from build123d import *

# Parameters (mm, degrees)
SKETCH1_W           = 23
SKETCH1_H           = 12
BOSS_EXTRUDE1_DEPTH = 4
SKETCH2_R           = 1.5
CUT_EXTRUDE1_DEPTH  = 10
SKETCH3_R           = 2
CUT_EXTRUDE2_DEPTH  = 14.57387196
CHAMFER1_SIZE       = 2


with BuildPart() as part:
    # Sketch1 → Boss-Extrude1 (new body)
    with BuildSketch(Plane(origin=(0, 0, 0), x_dir=(1, 0, 0), z_dir=(0, 1, 0))):
        Rectangle(SKETCH1_W, SKETCH1_H)
    extrude(amount=BOSS_EXTRUDE1_DEPTH)

    # Sketch2 → Cut-Extrude1 (cut)
    with BuildSketch(Plane(origin=(11.5, 0, 0), x_dir=(0, 0, -1), z_dir=(1, 0, 0))):
        with Locations((-4, 2)):
            Circle(SKETCH2_R)
        with Locations((4, 2)):
            Circle(SKETCH2_R)
    extrude(amount=-CUT_EXTRUDE1_DEPTH, mode=Mode.SUBTRACT)

    # Sketch3 → Cut-Extrude2 (cut, through all)
    with BuildSketch(Plane(origin=(0, 4, 0), x_dir=(1, 0, 0), z_dir=(0, 1, 0))):
        with Locations(Location((-5.5, 0, 0), (0, 0, 270))):
            Circle(SKETCH3_R)
    extrude(amount=-CUT_EXTRUDE2_DEPTH, mode=Mode.SUBTRACT)

    # Chamfer1
    chamfer1_edges = [part.edges().sort_by_distance(p)[0] for p in [
        (-11.5, 2, 6),
        (-11.5, 2, -6),
    ]]
    chamfer(chamfer1_edges, length=CHAMFER1_SIZE)


solid = part.part
Source: CAD feature listing. Evaluate the final solid. Frame: model axes, mm. A direction names the side the tool comes from. Give positions to 0.01 mm unless a question says otherwise; leave off trailing zeros. Write each loop counter-clockwise with the first axis right and the second up, starting at its lowest first coordinate (ties: lowest second). Pieces come first, ordered by that corner, then holes. Notation, with made-up numbers: (15, 51.25) -> (56, 51.25) arc R13 cw to (56, 65.25) -> close; hole circle Ø9 at (-11.75, -30). An arc over 180 degrees is marked (long way). Write item = value, one per line.
Q1. First-contact query: pin 1 (2 mm diameter, centred on y = 3, z = 4.5, fed in from -X). Flat tip, straight axial feed; report the tip coordinate or a pass-through.
Here are the results:
pin_1 = -11.5
Q2. Cut plane B-B on z = 0. Return loops of the section in (x, y).
Here are the results:
outline = (-11.5, 0) -> (-7.5, 0) -> (-7.5, 4) -> (-11.5, 4) -> close; (-3.5, 0) -> (11.5, 0) -> (11.5, 4) -> (-3.5, 4) -> close
Q3. Cut plane A-A on x = -5.5. Return loops of the section in (y, z), then the cut area to 3 significant figures.
Here are the results:
outline = (0, -6) -> (4, -6) -> (4, -2) -> (0, -2) -> close; (0, 2) -> (4, 2) -> (4, 6) -> (0, 6) -> close
area = 32.0 mm²
Q4. Cut plane C-C on y = 1.5. Return loops of the section in (x, z).
Here are the results:
outline = (-11.5, -4) -> (-9.5, -6) -> (11.5, -6) -> (11.5, -5.41) -> (1.5, -5.41) -> (1.5, -2.59) -> (11.5, -2.59) -> (11.5, 2.59) -> (1.5, 2.59) -> (1.5, 5.41) -> (11.5, 5.41) -> (11.5, 6) -> (-9.5, 6) -> (-11.5, 4) -> close; hole circle Ø4 at (-5.5, 0)
Q5. Mould query, pull axis Y, two halves, no side actions, for faces 3 (the face through (0, 4, 0)), 4 (the face through (1.5, 2, -4)), 5 (the face through (11.5, 2, 0)). Classes: +Y half, -Y half, draft (parallel to the pull), parting line (faces both ways), or undercut.
Here are the results:
face_3 = +Y half
face_4 = undercut
face_5 = draft
Q6. Line query: line 1 (Y direction, x = 7.5, z = -4); line 2 (X direction, y = 1.65, z = 0); line 3 (Z direction, x = 5.5, y = 1.65). Output: solid intervals per line, ascending. Write a range as from..to.
Here are the results:
line_1 = 0..0.5, 3.5..4
line_2 = -11.5..-7.5, -3.5..11.5
line_3 = -6..-5.46, -2.54..2.54, 5.46..6
Q7. Reachability of faces 1 (the face through (-7.452, 2.028, -0.434)), 2 (the face through (1.5, 2, 4)) from +Z, -Z, +X, -X, +Y, -Y: full face, straight path, thin tool, end or side. Return the list, or none.
Here are the results:
face_1 = +Y, -Y
face_2 = +X
Q8. Cut plane D-D on x = 5.75. Return loops of the section in (y, z), then the cut area to 3 significant figures.
Here are the results:
outline = (0, -6) -> (4, -6) -> (4, 6) -> (0, 6) -> close; hole circle Ø3 at (2, -4); hole circle Ø3 at (2, 4)
area = 33.9 mm²
